Solid Edge part; units mm, degrees
sketch "Sketch1" plane through (0, 0, 0) normal (0, -1, 0) x (1, 0, 0)
  line L0 (44, 17) -> (44, 0)
  line L1 (12, 0) -> (44, 0)
  line L2 (12, 0) -> (12, 32)
  line L3 (12, 32) -> (29, 32)
  arc A0 (29, 32) -> (44, 17) centre (29, 17) cw
extrude "Protrusion1" add sketch "Sketch1" along normal blind 25
sketch "Sketch2" plane through (0, 0, 0) normal (0, -1, 0) x (1, 0, 0)
  arc A0 (44, 0) -> (12, -32) centre (12, 0) cw
  line L0 (12, -32) -> (-40, -32)
  line L1 (-40, -32) -> (-40, 40)
  line L2 (-40, 40) -> (-12, 40)
  line L3 (-12, 40) -> (-12, 0)
  arc A1 (12, 0) -> (-12, 0) centre (0, 0) cw
  line L4 (12, 0) -> (44, 0)
extrude "ExtrudedProtrusion_2" add sketch "Sketch2" along normal blind 80
sketch "Sketch3" plane through (2, -80, 4) normal (0, -1, 0) x (1, 0, 0)
  line L0 (-14, 12) -> (-42, 12)
  line L1 (-42, 12) -> (-42, 28)
  line L2 (-42, 28) -> (-14, 28)
  line L3 (-14, 28) -> (-14, 12)
extrude "ExtrudedCutout_1" cut sketch "Sketch3" against normal blind 8
sketch "Sketch4" plane through (-40, -40, 4) normal (-1, 0, 0) x (0, -1, 0)
  line L0 (0, -4) -> (0, 11)
  line L1 (0, 11) -> (12, 36)
  line L2 (0, 36) -> (12, 36)
  line L3 (-40, 36) -> (0, 36)
  line L4 (-40, 36) -> (-40, -4)
  line L5 (-40, -4) -> (-40, -36)
  line L6 (-40, -36) -> (0, -36)
  line L7 (0, -36) -> (0, -4)
extrude "ExtrudedCutout_2" cut sketch "Sketch4" against normal blind 52
Could you check a few things on this model? Use its own coordinates, in mm. A direction names the side the tool comes from. Round coordinates to 2 decimals unless told otherwise and drop trailing zeros. Write each loop counter-clockwise with the first axis right and the second up, starting at its lowest first coordinate (ties: lowest second). Pieces come first, ordered by that corner, then holes. Notation, with made-up numbers: M -1,13 L 43,13 A19 ccw 43,37 Z; hole C 8,74.5 d6. An arc over 180 degrees is marked long. Answer in a Markdown table with one row per item. Add a question column.
Q1. Imagine slicing it at C-C (x = 0). Please give me the cut outline in (y, z).
Q2. Imagine slicing it at A-A (z = 26). Please give me the cut outline in (x, y).
Q3. Will these pins go through, and if not, where does the flat tip stop? pin 1 Ø13 at (x, z) = (-29.5, 25) entering from -Y; pin 2 Ø12 at (x, y) = (-28, -40) entering from +Z; pin 3 Ø1.5 at (x, y) = (13.5, -18) entering from +Z; pin 4 Ø12 at (x, z) = (3.5, 24.5) entering from +Y.
Q4. If we mould it in two halves opening along Z, with no side actions, what happens to faces 4 (the flat face through (-26, -72, 24)), 5 (the flat face through (-26, -66, 40)), 6 (the cylindrical face through (34.87, -39.44, -22.38))? For each: +Z half, -Z half, draft (parallel to the pull), parting line (faces both ways), or undercut.
Q5. If I drill on line 1 (X direction, y = -56, z = 15); line 2 (X direction, y = -48.5, z = -1.5); line 3 (Y direction, x = -21.5, z = -17.5), over which ranges is the centre line in solid material (lowest first)? Write a range as from..to.
Q6. Imagine slicing it at B-B (y = -57). Please give me the cut outline in (x, z).
Q7. On a 3-axis mill with a long thin cutter (end or side, diameter ignored), from which of +Z, -Z, +X, -X, +Y, -Y can I reach the whole of each face in a straight line? I mean faces 1 (the flat face through (28, -25, 16)), 2 (the flat face through (-26, -76, 16)), 3 (the flat face through (-12, -60, 20)). Say none if no direction works.
Q8. Imagine slicing it at D-D (z = -26). Please give me the cut outline in (x, y), then the cut area to 3 significant figures.
Values:
| question | item | result |
|---|---|---|
| 1 | outline | M -80,-32 L -40,-32 L -40,-12 L -80,-12 Z |
| 2 | outline | M -40,-72 L -12,-72 L -12,-45.28 L -40,-45.28 Z; M 12,-25 L 41,-25 L 41,0 L 12,0 Z |
| 3 | pin 1 | y = -72 |
| 3 | pin 2 | z = 27.5 |
| 3 | pin 3 | z = 32 |
| 3 | pin 4 | through |
| 4 | face 4 | undercut |
| 4 | face 5 | +Z half |
| 4 | face 6 | -Z half |
| 5 | line 1 | -40..-12 |
| 5 | line 2 | -40..-11.91, 11.91..43.96 |
| 5 | line 3 | -80..-40 |
| 6 | outline | M -40,-32 L 12,-32 A32 ccw 44,0 L 12,0 A12 cw -12,0 L -12,40 L -40,40 Z |
| 7 | face 1 | +Z, +X, -X, -Y |
| 7 | face 2 | +X, -X, -Y |
| 7 | face 3 | +Z, +X, +Y, -Y |
| 8 | outline | M -40,-80 L 30.65,-80 L 30.65,0 L 12,0 L 12,-40 L -40,-40 Z |
| 8 | area | 3,570 mm^2 |
